from build123d import *

# Parameters (mm, degrees)
SKETCH1_W           = 11.6
SKETCH1_H           = 10.5
BOSS_EXTRUDE1_DEPTH = 4.25
SKETCH2_W           = 10.6
SKETCH2_H           = 0.5
CUT_EXTRUDE1_DEPTH  = 12.552164299
SKETCH3_W           = 0.7
SKETCH3_H           = 0.25
BOSS_EXTRUDE2_DEPTH = 4.5


with BuildPart() as part:
    # Sketch1 → Boss-Extrude1 (new, symmetric)
    with BuildSketch(Plane.XY):
        Rectangle(SKETCH1_W, SKETCH1_H)
    extrude(amount=BOSS_EXTRUDE1_DEPTH, both=True)

    # Sketch2 → Cut-Extrude1 (cut, through all)
    with BuildSketch(Plane.XY.offset(4.25)):
        with Locations((0, -5)):
            Rectangle(SKETCH2_W, SKETCH2_H)
    extrude(amount=-CUT_EXTRUDE1_DEPTH, mode=Mode.SUBTRACT)

    # Sketch3 → Boss-Extrude2 (add)
    with BuildSketch(Plane(origin=(0, -4.75, 0), x_dir=(-1, 0, 0), z_dir=(0, -1, 0))):
        with Locations((0, -2.25)):
            Rectangle(SKETCH3_W, SKETCH3_H)
        with Locations((2.54, -2.25)):
            Rectangle(SKETCH3_W, SKETCH3_H)
        with Locations((-2.54, -2.25)):
            Rectangle(SKETCH3_W, SKETCH3_H)
    extrude(amount=BOSS_EXTRUDE2_DEPTH)


solid = part.part
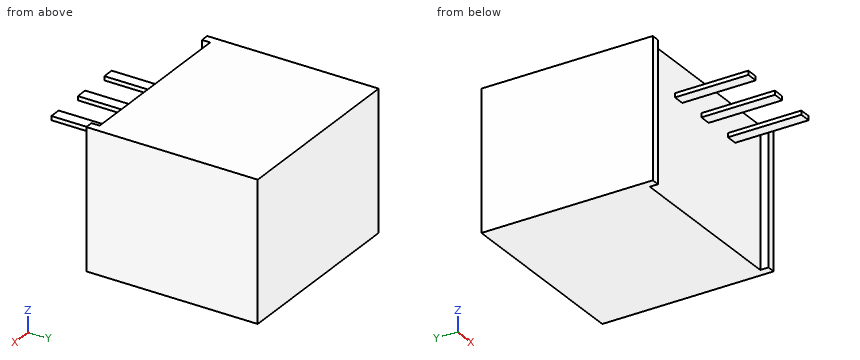
Could you check a few things on this model? Use its own coordinates, in mm. Give positions to 0.01 mm unless a question says otherwise; leave off trailing zeros. Order: outer loops, then holes, each group sorted by start corner. A loop starts at its lowest first (then second) coordinate and runs counter-clockwise, first axis right, second up. Notation, with made-up numbers: (17, 73) - (48, 73) arc R16 cw to (48, 87) - close; hole circle Ø5 at (39, 45.25). An arc over 180 degrees is marked (long way). One line per item, written item: value. Start each with the question number.
1. For P1, Ø0.8, axis at x = 2.5, y = -8, coming from the -Z side (3 decimals); P2, Ø2, axis at x = 0.5, z = 3.5, coming from the -Y side; P3, Ø0.8, axis at x = 0, y = -6, coming from the +Z side (3 decimals), each with a flat end and sliding along its axis, tell me the tip position at first contact or that it passes through.
2. If I drill on probe 1 along Y at (x, z) = (4, -1.5); probe 2 along Z at (x, y) = (-2.75, -7.25) (3 decimals), over which ranges is the centre line in solid material (lowest first)?
3. Imagine slicing it at C-C on x = -2.5. List the corners of the cut face in (y, z) for me (3 decimals).
4. Imagine slicing it at A-A on y = -8. List the corners of the cut face in (x, z) for me (3 decimals).
5. Imagine slicing it at D-D on x = 4. List the corners of the cut face in (y, z) for me.
6. Imagine slicing it at B-B on z = -1.25. List the corners of the cut face in (x, y) for me.
Values:
1. P1: z = 2.125
1. P2: y = -4.75
1. P3: z = 2.375
2. probe 1: -4.75 to 5.25
2. probe 2: 2.125 to 2.375
3. outline: (-9.25, 2.125) - (-4.75, 2.125) - (-4.75, -4.25) - (5.25, -4.25) - (5.25, 4.25) - (-4.75, 4.25) - (-4.75, 2.375) - (-9.25, 2.375) - close
4. outline: (-2.89, 2.125) - (-2.19, 2.125) - (-2.19, 2.375) - (-2.89, 2.375) - close; (-0.35, 2.125) - (0.35, 2.125) - (0.35, 2.375) - (-0.35, 2.375) - close; (2.19, 2.125) - (2.89, 2.125) - (2.89, 2.375) - (2.19, 2.375) - close
5. outline: (-4.75, -4.25) - (5.25, -4.25) - (5.25, 4.25) - (-4.75, 4.25) - close
6. outline: (-5.8, -5.25) - (-5.3, -5.25) - (-5.3, -4.75) - (5.3, -4.75) - (5.3, -5.25) - (5.8, -5.25) - (5.8, 5.25) - (-5.8, 5.25) - close
